from build123d import *

# Parameters (mm, degrees)
SKETCH1_W          = 46.99
SKETCH1_H          = 43.18
EXTRUDE1_DEPTH     = 67.818
FILLET2_R          = 1.27
SKETCH2_R          = 15.875
SKETCH2_R_2        = 12.065
EXTRUDE2_DEPTH     = 2.54
SKETCH3_R          = 1.0795
CUT_EXTRUDE1_DEPTH = 2.54


with BuildPart() as part:
    # Sketch1 → Extrude1 (new body)
    with BuildSketch(Plane.XY):
        Rectangle(SKETCH1_W, SKETCH1_H)
    extrude(amount=EXTRUDE1_DEPTH)

    # Fillet2
    fillet2_edges = [part.edges().sort_by_distance(p)[0] for p in [
        (23.495, 0, 67.818),
        (0, 21.59, 67.818),
        (-23.495, 0, 67.818),
        (0, 21.59, 0),
        (23.495, 0, 0),
        (0, -21.59, 0),
        (-23.495, 0, 0),
        (0, -21.59, 67.818),
        (-23.495, 21.59, 33.909),
        (23.495, 21.59, 33.909),
        (23.495, -21.59, 33.909),
        (-23.495, -21.59, 33.909),
    ]]
    fillet(fillet2_edges, radius=FILLET2_R)

    # Sketch2 → Extrude2 (add)
    with BuildSketch(Plane.XY.offset(67.818)):
        Circle(SKETCH2_R)
        Circle(SKETCH2_R_2, mode=Mode.SUBTRACT)
    extrude(amount=EXTRUDE2_DEPTH)

    # Sketch3 → Cut-Extrude1 (cut)
    with BuildSketch(Plane.XZ.offset(21.59)):
        with Locations((-10.922, 39.1795)):
            Circle(SKETCH3_R)
        with Locations((10.795, 39.1795)):
            Circle(SKETCH3_R)
    extrude(amount=-CUT_EXTRUDE1_DEPTH, mode=Mode.SUBTRACT)


solid = part.part
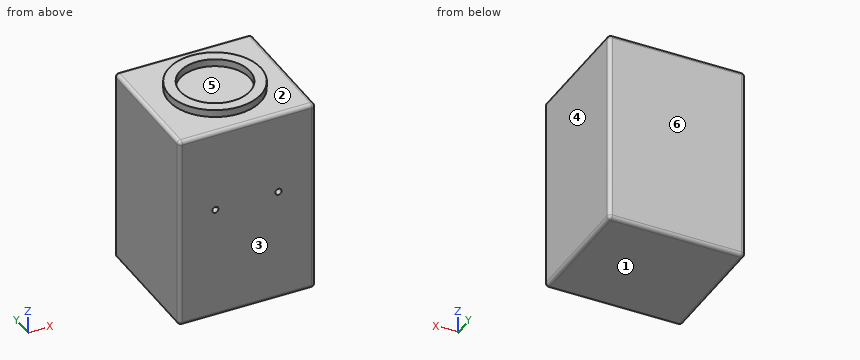
The listing builds one solid part. Answer for the finished solid, in the listing's coordinates (mm). Face numbers are marked on the shaded views. A direction names the side the tool comes from. Round coordinates to 2 decimals unless told otherwise and drop trailing zeros. Write each loop counter-clockwise with the first axis right and the second up, starting at its lowest first coordinate (ties: lowest second). Pieces come first, ordered by that corner, then holes. Notation, with made-up numbers: M 87.5,-9.75 L 108.5,-9.75 A26 ccw 108.5,23.25 Z; hole C -3.75,43 d4. An arc over 180 degrees is marked long. Write each question's results on one line, items separated by ' | '. Start each with the question number.
(1) For the marked faces 1 and 2, determine the directions among +Z, -Z, +X, -X, +Y, -Y from which every point of the face is accessible in a straight line to the end or side of a thin tool.
(2) The part is cut by section D-D, the plane y = 18. Write down the section's boundary in (x, z) (3 decimals).
(3) The part is cut by section B-B, the plane y = 0. Write down the section's boundary in (x, z) (3 decimals), and give its area (3 significant figures).
(4) Determine the mould class of the marked faces 3, 4, 5 and 6 for opening direction Y: +Y half, -Y half, draft (parallel to the pull), parting line (faces both ways), or undercut.
(5) Find the intervals of material crossed by line 1 (Z direction, x = -17, y = -11.5), in increasing order.
(6) The part is cut by section A-A, the plane x = 17.5. Write down the section's boundary in (y, z), and give its area (3 significant figures).
(7) The part is cut by section C-C, the plane x = 0. Write down the section's boundary in (y, z) (3 decimals).
(8) Each of these flat-tipped pins is pushed along its axis until it touches: P1, Ø1.1, axis at x = 11, z = 39.5, coming from the -Y side; P2, Ø8, axis at x = 3.5, y = 6, coming from the +Z side. Where does it stop, or does it pass through?
Worked answers:
1) face 1: -Z, +X, -X, +Y, -Y | face 2: +Z
2) outline: M -23.495,1.27 A1.27 ccw -22.225,0 L 22.225,0 A1.27 ccw 23.495,1.27 L 23.495,66.548 A1.27 ccw 22.225,67.818 L -22.225,67.818 A1.27 ccw -23.495,66.548 Z
3) outline: M -23.495,1.27 A1.27 ccw -22.225,0 L 22.225,0 A1.27 ccw 23.495,1.27 L 23.495,66.548 A1.27 ccw 22.225,67.818 L 15.875,67.818 L 15.875,70.358 L 12.065,70.358 L 12.065,67.818 L -12.065,67.818 L -12.065,70.358 L -15.875,70.358 L -15.875,67.818 L -22.225,67.818 A1.27 ccw -23.495,66.548 Z | area: 3,200 mm²
4) face 3: -Y half | face 4: draft | face 5: undercut | face 6: +Y half
5) line 1: z = 0 to 67.82
6) outline: M -21.59,1.27 A1.27 ccw -20.32,0 L 20.32,0 A1.27 ccw 21.59,1.27 L 21.59,66.55 A1.27 ccw 20.32,67.82 L -20.32,67.82 A1.27 ccw -21.59,66.55 Z | area: 2,930 mm²
7) outline: M -21.59,1.27 A1.27 ccw -20.32,0 L 20.32,0 A1.27 ccw 21.59,1.27 L 21.59,66.548 A1.27 ccw 20.32,67.818 L 15.875,67.818 L 15.875,70.358 L 12.065,70.358 L 12.065,67.818 L -12.065,67.818 L -12.065,70.358 L -15.875,70.358 L -15.875,67.818 L -20.32,67.818 A1.27 ccw -21.59,66.548 Z
8) P1: stops at y = -19.05 | P2: stops at z = 67.82
